For this review, take the finished solid that the model builds, in its own axes (mm). A direction names the side the tool comes from. Round coordinates to 2 decimals unless told otherwise and drop trailing zeros. Loops run counter-clockwise (first coordinate to the right, second up) from the corner with the lowest first, then second, coordinate; pieces in that order, holes last.
1) Take a section at C-C (z = 22.5). State the section outline as (x, y) points, then the cut area to 3 significant figures.
2) Wall thickness on L1, parallel to Z at x = -13.5, y = -50; L2, parallel to Z at x = -15.5, y = 45.5; L3, parallel to X at y = 62, z = 25.5: over which ranges is each line inside the solid? List them lowest first.
3) Tool access review of faces 4 (the flat face through (-54.6, 0.8, 15)), 5 (the flat face through (-15, 0.8, 54.6)), 6 (the flat face through (-63.033, -1, 5)), 7 (the flat face through (-34.32, -43.59, 34.47)), 8 (the flat face through (-24, -70, 25)): name each direction out of +Z, -Z, +X, -X, +Y, -Y from which nothing blocks a thin tool from reaching the whole face with its end or side.
4) Mouldability with a two-part tool opening along Y and no side actions: class faces 1 (the flat face through (0, -1, 32)), 2 (the flat face through (-32, -30.854, 33)), 3 (the flat face through (-24, 70, 25)) as pulls with the +Y half, pulls with the -Y half, needs draft (parallel to the pull), parting line crosses it, or undercut.
5) Take a section at B-B (x = -43). State the section outline as (y, z) points.
6) Take a section at A-A (y = 8.5). State the section outline as (x, z) points.
7) Insertion check: pin 1 (4 mm diameter, centred on y = -37, z = 40.5, fed in from -X); pin 2 (8 mm diameter, centred on y = -45.5, z = 35, fed in from -X); pin 3 (21.5 mm diameter, centred on x = -35.5, z = 39.5, fed in from -Y); pin 4 (1.5 mm diameter, centred on y = 32, z = 47.5, fed in from -X). Each pin has a flat end and moves straight along its axis. Give the tip position at first contact, or say it passes through.
```python
from build123d import *

# Parameters (mm, degrees)
PAD_DEPTH       = 70
PAD_DEPTH_BACK  = 70
SKETCH001_W     = 56
SKETCH001_H     = 110
POCKET_DEPTH    = 5
SKETCH002_W     = 55
SKETCH002_H     = 85
POCKET001_DEPTH = 1
SKETCH003_R     = 7.812733
PAD001_DEPTH    = 2


with BuildPart() as part:
    # Sketch → Pad (new body, two sides)
    with BuildSketch(Plane.XZ) as pad_sk:
        Polygon((-63.033008589, 0), (-63.033008589, 10), (-10, 63.033008589), (0, 63.033008589), (0, 0), align=None)
    extrude(amount=PAD_DEPTH)
    extrude(pad_sk.sketch, amount=-PAD_DEPTH_BACK)

    # Sketch001 (on Face2 of Pad) → Pocket (cut)
    with BuildSketch(Plane(origin=(-36.5165042945, 0, 36.5165042945), x_dir=(-0.7071067812, 0, -0.7071067812), z_dir=(-0.7071067812, 0, 0.7071067812))):
        Rectangle(SKETCH001_W, SKETCH001_H)
    extrude(amount=-POCKET_DEPTH, mode=Mode.SUBTRACT)

    # Sketch002 (on Face12 of Pocket) → Pocket001 (cut)
    with BuildSketch(Plane(origin=(-32.9809703886, 0, 32.9809703886), x_dir=(-0.7071067812, 0, -0.7071067812), z_dir=(-0.7071067812, 0, 0.7071067812))):
        with Locations((0, -11.6462930524)):
            Rectangle(SKETCH002_W, SKETCH002_H)
    extrude(amount=-POCKET001_DEPTH, mode=Mode.SUBTRACT)

    # Sketch003 (on Face12 of Pocket001) → Pad001 (join)
    with BuildSketch(Plane(origin=(-32.9809703886, 0, 32.9809703886), x_dir=(-0.7071067812, 0, -0.7071067812), z_dir=(-0.7071067812, 0, 0.7071067812))):
        with Locations((0, 43.476822)):
            Circle(SKETCH003_R)
    extrude(amount=PAD001_DEPTH)


solid = part.part
```
Response:
1. outline: (-50.53, -70) - (0, -70) - (0, 70) - (-50.53, 70) - (-50.53, 55) - (-43.46, 55) - (-43.46, 54.15) - (-42.05, 54.15) - (-42.05, -30.85) - (-43.46, -30.85) - (-43.46, -55) - (-50.53, -55) - close
1. area: 6,180 mm2
2. L1: z = 0 to 52.46, 53.1 to 59.53
2. L2: z = 0 to 49.05, 55.1 to 57.53
2. L3: x = -47.53 to 0
3. face 4: +Z
3. face 5: -X
3. face 6: +Z, -Z, -X, +Y, -Y
3. face 7: +Z, -X
3. face 8: +Z, -Z, +X, -X, -Y
4. face 1: needs draft
4. face 2: undercut
4. face 3: pulls with the +Y half
5. outline: (-70, 0) - (70, 0) - (70, 30.03) - (55, 30.03) - (55, 22.96) - (54.15, 22.96) - (54.15, 21.55) - (-30.85, 21.55) - (-30.85, 22.96) - (-55, 22.96) - (-55, 30.03) - (-70, 30.03) - close
6. outline: (-63.03, 0) - (0, 0) - (0, 63.03) - (-10, 63.03) - (-16.72, 56.32) - (-13.18, 52.78) - (-13.54, 52.43) - (-12.83, 51.72) - (-51.72, 12.83) - (-52.43, 13.54) - (-52.78, 13.18) - (-56.32, 16.72) - (-63.03, 10) - close
7. pin 1: stops at x = -27.46
7. pin 2: stops at x = -37.79
7. pin 3: stops at y = -70
7. pin 4: stops at x = -17.8
